from build123d import *

# Parameters (mm, degrees)
CUT_EXTRUDE_1_DEPTH      = 0.3
PATTERN_CIRCULAR_1_COUNT = 2
PATTERN_CIRCULAR_1_ANGLE = 90


with BuildPart() as part:
    # 草图1 → 旋转3 (revolve)
    with BuildSketch(Plane(origin=(0, 0, 0), x_dir=(0, 0, -1), z_dir=(1, 0, 0)), mode=Mode.PRIVATE) as revolve_3_sk:
        with BuildLine():
            ThreePointArc((1.375, -1.2), (1.657842712, -1.082842712), (1.775, -0.8))
            Line((1.775, -0.8), (1.775, -0.649888064))
            ThreePointArc((1.775, -0.649888064), (1.709909462, -0.431174433), (1.535821739, -0.283641742))
            ThreePointArc((1.535821739, -0.283641742), (0.784373982, -0.052678823), (0, 0))
            Line((0, 0), (0, -13.2))
            Line((0, -13.2), (0.95, -13.2))
            Line((0.95, -13.2), (0.95, -1.2))
            Line((0.95, -1.2), (1.375, -1.2))
        make_face()
    revolve(revolve_3_sk.sketch.rotate(Axis((0, 0, 0), (0, -1, 0)), 180), axis=Axis((0, 0, 0), (0, -1, 0)))

    # 草图5 → 切除-拉伸1 (cut, symmetric)
    with BuildSketch(Plane(origin=(0, 0, 0), x_dir=(0, 0, -1), z_dir=(1, 0, 0))):
        Polygon((-1.8, 0.488536713), (-0.5, -0.8838523), (0.5, -0.8838523), (1.8, 0.488536713), align=None)
    cut_extrude_1 = extrude(amount=CUT_EXTRUDE_1_DEPTH, both=True, mode=Mode.SUBTRACT)

    # 阵列(圆周)1: 切除-拉伸1 ×2 about axis
    pattern_circular_1_axis = Axis((0, 0, 0), (0, -1, 0))
    for i in range(1, PATTERN_CIRCULAR_1_COUNT):
        add(cut_extrude_1.rotate(pattern_circular_1_axis, i * PATTERN_CIRCULAR_1_ANGLE / (PATTERN_CIRCULAR_1_COUNT - 1)), mode=Mode.SUBTRACT)


solid = part.part
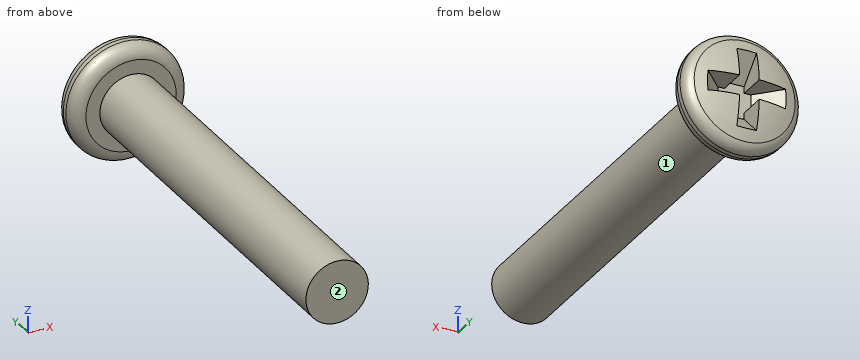
Verification items for the finished model (mm, model axes). Face numbers are marked on the shaded views. Coordinates: 2 decimals unless noted, no trailing zeros. Order: outer loops, then holes, each group sorted by start corner. A loop starts at its lowest first (then second) coordinate and runs counter-clockwise, first axis right, second up. Notation, with made-up numbers: M 72.5,31 L 76.5,31 A4 cw 76.5,38 Z; hole C -10,54.5 d8. An arc over 180 degrees is marked long. One line per item, written item: value. Start each with the question number.
Item 1: Depth check by flat-ended pin: P1, Ø1, axis at y = -0.5, z = -1, coming from the -X side; P2, Ø2, axis at y = -10.5, z = 1, coming from the +X side; P3, Ø1.5, axis at x = 0.5, y = -8.5, coming from the +Z side. Enter the tip coordinate at first touch or a pass-through.
Item 2: Thickness scan on probe 1 along Z at (x, y) = (-0.05, -8.75); probe 2 along Y at (x, z) = (-0.7, 0.25). Record the ranges inside material, lowest first.
Item 3: Sectioned sample at A-A on y = -8.5. Record the cut outline in (x, z), then the cut area to 3 significant figures.
Item 4: Mould release check, pull along X, two halves, no side actions. Record for the marked faces 1 and 2: pulls with the +X half, pulls with the -X half, needs draft (parallel to the pull), parting line crosses it, or undercut.
Calculated:
1. P1: x = -1.7
1. P2: x = 0.95
1. P3: z = 0.95
2. probe 1: -0.95 to 0.95
2. probe 2: -13.2 to -0.67
3. outline: C 0,0 d1.9
3. area: 2.84 mm^2
4. face 1: parting line crosses it
4. face 2: needs draft
